Part model, mm, in its own coordinate system. Coordinates: 2 decimals unless noted, no trailing zeros. Order: outer loops, then holes, each group sorted by start corner. A loop starts at its lowest first (then second) coordinate and runs counter-clockwise, first axis right, second up. Notation, with made-up numbers: (-1.75, 41) - (16.25, 41) arc R10 cw to (16.25, 49) - close; hole circle Ø9 at (3, 40). An arc over 180 degrees is marked (long way). Use a Markdown table: item, result. Add a question column.
1) Saw through at B-B on y = -177.5. List the corners of the cut face in (x, z), then the cut area to 3 significant figures.
2) Saw through at A-A on y = -352. List the corners of the cut face in (x, z).
3) Wall check: L1, parallel to X at y = -465, z = -149.25; L2, parallel to X at y = -250, z = 202.5; L3, parallel to X at y = -432, z = 202. Give the ranges that are in metal, low to high. Write a range as [from, to].
4) Drop flat-ended pins along their axis: P1, Ø5, axis at x = -396.37, y = -450, coming from the +Z side; P2, Ø2.5, axis at x = 333.63, y = -265, coming from the -Z side; P3, Ø22, axis at x = 343.5, z = 200, coming from the -Y side; P4, Ø21.5, axis at x = -92, z = 261, coming from the -Y side. Give the stop position or say it passes through.
5) Saw through at C-C on z = 13.5. List the corners of the cut face in (x, y), then the cut area to 3 significant figures.
```python
from build123d import *

# Parameters (mm, degrees)
SKETCH_1_W      = 750
SKETCH_1_H      = 519.2
SKETCH_1_W_2    = 710
SKETCH_1_H_2    = 479.2
EXTRUDE_1_DEPTH = 20
SKETCH_2_W      = 20
SKETCH_2_H      = 20
EXTRUDE_2_DEPTH = 470
SKETCH_6_W      = 20
SKETCH_6_H      = 20
EXTRUDE_4_DEPTH = 270
SKETCH_4_R      = 1.6
EXTRUDE1_DEPTH  = 30
SKETCH_7_R      = 1.5
EXTRUDE2_DEPTH  = 30
SKETCH1_R       = 8
EXTRUDE3_DEPTH  = 20


with BuildPart() as part:
    # 草图1 → 凸台-拉伸1 (new body)
    with BuildSketch(Plane(origin=(0, 0, 0), x_dir=(1, 0, 0), z_dir=(0, 1, 0))):
        with Locations((-25.365803698, -25.141816005)):
            Rectangle(SKETCH_1_W, SKETCH_1_H)
        with Locations((-25.365803698, -25.141816005)):
            Rectangle(SKETCH_1_W_2, SKETCH_1_H_2, mode=Mode.SUBTRACT)
    extrude(amount=EXTRUDE_1_DEPTH)

    # 草图2 → 凸台-拉伸2 (add)
    with BuildSketch(Plane.XZ):
        with Locations((-390.365803698, 202.741816005)):
            Rectangle(SKETCH_2_W, SKETCH_2_H)
    extrude_2 = extrude(amount=EXTRUDE_2_DEPTH)

    # 草图6 → 凸台-拉伸4 (add)
    with BuildSketch(Plane.XZ):
        with Locations((339.634196302, -152.458183995)):
            Rectangle(SKETCH_6_W, SKETCH_6_H)
    extrude_4 = extrude(amount=EXTRUDE_4_DEPTH)

    # 草图4 → Extrude1 (cut)
    with BuildSketch(Plane.XY.offset(212.741816005)):
        with Locations((-396.365803698, -465)):
            Circle(SKETCH_4_R)
        with Locations((-384.365803698, -465)):
            Circle(SKETCH_4_R)
        with Locations((-396.365803698, -450)):
            Circle(SKETCH_4_R)
        with Locations((-384.365803698, -450)):
            Circle(SKETCH_4_R)
    extrude1 = extrude(amount=-EXTRUDE1_DEPTH, mode=Mode.SUBTRACT)

    # 草图7 → Extrude2 (cut)
    with BuildSketch(Plane(origin=(0, 0, -162.458183995), x_dir=(-1, 0, 0), z_dir=(0, 0, -1))):
        with Locations((-345.634196302, -265)):
            Circle(SKETCH_7_R)
        with Locations((-333.634196302, -265)):
            Circle(SKETCH_7_R)
        with Locations((-345.634196302, -250)):
            Circle(SKETCH_7_R)
        with Locations((-333.634196302, -250)):
            Circle(SKETCH_7_R)
    extrude2 = extrude(amount=-EXTRUDE2_DEPTH, mode=Mode.SUBTRACT)

    # Mirror1: 凸台-拉伸2, 凸台-拉伸4, Extrude1, Extrude2 across plane
    add(extrude_2.mirror(Plane.XY.offset(25.141816005)))
    add(extrude_4.mirror(Plane.XY.offset(25.141816005)))
    add(extrude1.mirror(Plane.XY.offset(25.141816005)), mode=Mode.SUBTRACT)
    add(extrude2.mirror(Plane.XY.offset(25.141816005)), mode=Mode.SUBTRACT)

    # Sketch1 → Extrude3 (cut)
    with BuildSketch(Plane(origin=(0, 20, 0), x_dir=(1, 0, 0), z_dir=(0, 1, 0))):
        with Locations((-25.365803698, 224.458183995)):
            Circle(SKETCH1_R)
        with Locations((-25.365803698, -274.741816005)):
            Circle(SKETCH1_R)
    extrude(amount=-EXTRUDE3_DEPTH, mode=Mode.SUBTRACT)


solid = part.part
```
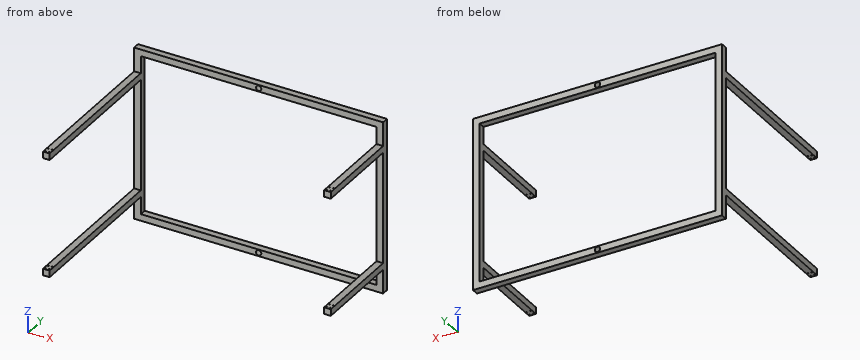
Results are:
| question | item | result |
|---|---|---|
| 1 | outline | (-400.37, -162.46) - (-380.37, -162.46) - (-380.37, -142.46) - (-400.37, -142.46) - close; (-400.37, 192.74) - (-380.37, 192.74) - (-380.37, 212.74) - (-400.37, 212.74) - close; (329.63, -162.46) - (349.63, -162.46) - (349.63, -142.46) - (329.63, -142.46) - close; (329.63, 192.74) - (349.63, 192.74) - (349.63, 212.74) - (329.63, 212.74) - close |
| 1 | area | 1,600 mm2 |
| 2 | outline | (-400.37, -162.46) - (-380.37, -162.46) - (-380.37, -142.46) - (-400.37, -142.46) - close; (-400.37, 192.74) - (-380.37, 192.74) - (-380.37, 212.74) - (-400.37, 212.74) - close |
| 3 | L1 | [-400.37, -397.97], [-394.77, -385.97], [-382.77, -380.37] |
| 3 | L2 | [-400.37, -380.37], [329.63, 332.13], [335.13, 344.13], [347.13, 349.63] |
| 3 | L3 | [-400.37, -380.37] |
| 4 | P1 | z = 212.74 |
| 4 | P2 | through |
| 4 | P3 | y = -270 |
| 4 | P4 | y = 0 |
| 5 | outline | (-400.37, 0) - (-380.37, 0) - (-380.37, 20) - (-400.37, 20) - close; (329.63, 0) - (349.63, 0) - (349.63, 20) - (329.63, 20) - close |
| 5 | area | 800 mm2 |
